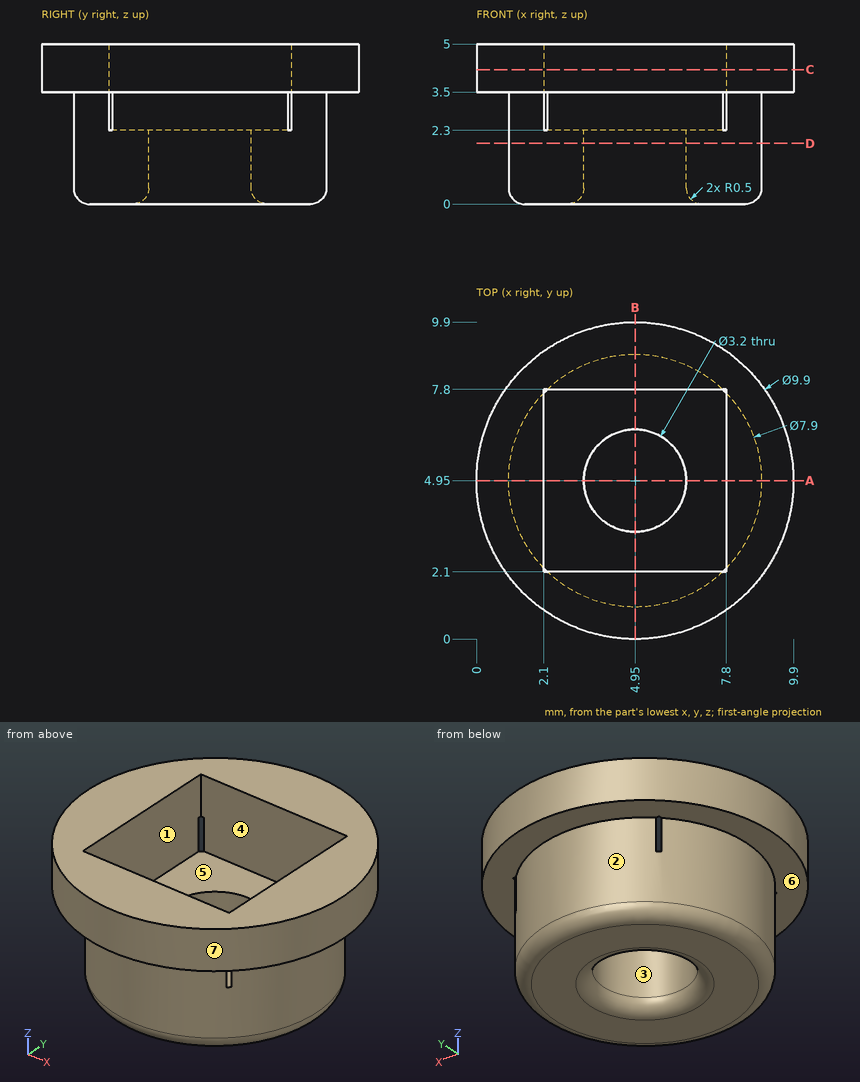
Check sheet for the drawn part. Datum: minimum x, y, z corner. Units: mm. A direction names the side the tool comes from. Give positions to 0.01 mm unless a question says otherwise; leave off trailing zeros. Loops run counter-clockwise (first coordinate to the right, second up) from the corner with the lowest first, then second, coordinate; pieces in that order, holes last. Notation, with made-up numbers: M 18,79 L 28,79 A20 ccw 28,94 Z; hole C 53,49.5 d6. An arc over 180 degrees is marked long. Return JSON: item names as keys, results as strings.
1) Mould release check, pull along X, two halves, no side actions. Record for the marked faces 4, 5, 6 and 7: released by +X, released by -X, zero draft, split by the parting line, or undercut.
Findings:
{"face 4": "undercut", "face 5": "undercut", "face 6": "zero draft", "face 7": "split by the parting line"}
2) Section check C-C, the plane z = 4.2. Enter the section's corners in (x, y), and give its area (3 significant figures).
Findings:
{"outline": "C 4.95,4.95 d9.9; hole M 2.1,2.1 L 7.8,2.1 L 7.8,7.8 L 2.1,7.8 Z", "area": "44.5 mm2"}
3) Material ranges on L1, parallel to X at y = 4.95, z = 1.95; L2, parallel to Z at x = 3, y = 6.5, recorded low to high. Write a range as [from, to].
Findings:
{"L1": "x = [1, 3.35], [6.55, 8.9]", "L2": "z = [0, 2.3]"}
4) Gauge pin test, flat ends, axial feed: P1, Ø2, axis at x = 4, z = 3.5, coming from the +Y side; P2, Ø3, axis at y = 2, z = 3.5, coming from the -X side; P3, Ø1, axis at x = 5, z = 2.5, coming from the +Y side; P4, Ø1.4, axis at y = 4, z = 3.5, coming from the +X side. Record the tip position at first contact, or that the pin passes through.
Findings:
{"P1": "stops at y = 9.9", "P2": "stops at x = 0.22", "P3": "stops at y = 8.9", "P4": "stops at x = 9.89"}
5) Section check D-D, the plane z = 1.9. Enter the section's corners in (x, y), and give its area (3 significant figures).
Findings:
{"outline": "C 4.95,4.95 d7.9; hole C 4.95,4.95 d3.2", "area": "41.0 mm2"}
6) Tool access check on the marked faces 1, 2 and 3. Record the directions out of +Z, -Z, +X, -X, +Y, -Y that give a thin tool (end or side, any length) a straight path to the whole face; none if there is none.
Findings:
{"face 1": "+Z", "face 2": "-Z", "face 3": "+Z, -Z"}
7) Section check A-A, the plane y = 4.95. Enter the section's corners in (x, z), and give its area (3 significant figures).
Findings:
{"outline": "M 0,3.5 L 1,3.5 L 1,0.5 A0.5 ccw 1.5,0 L 2.85,0 A0.5 ccw 3.35,0.5 L 3.35,2.3 L 2.1,2.3 L 2.1,5 L 0,5 Z; M 6.55,0.5 A0.5 ccw 7.05,0 L 8.4,0 A0.5 ccw 8.9,0.5 L 8.9,3.5 L 9.9,3.5 L 9.9,5 L 7.8,5 L 7.8,2.3 L 6.55,2.3 Z", "area": "19.5 mm2"}
